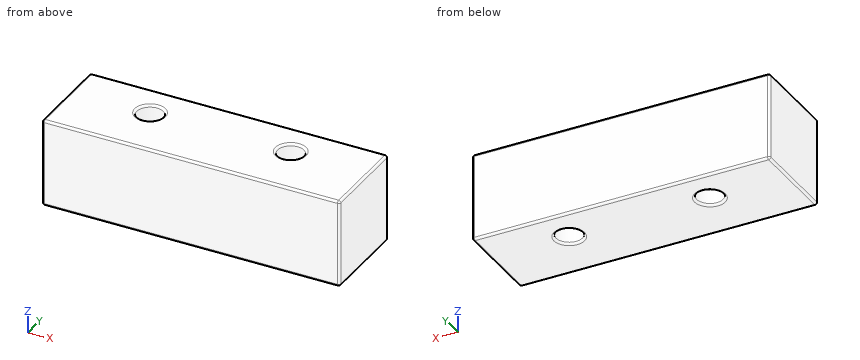
```python
from build123d import *

# Parameters (mm, degrees)
SKETCH1_W           = 67.684274796
SKETCH1_H           = 20.635526277
SKETCH1_R           = 3
BOSS_EXTRUDE1_DEPTH = 20
FILLET1_R           = 0.5


with BuildPart() as part:
    # Sketch1 → Boss-Extrude1 (new body)
    with BuildSketch(Plane.XY):
        with Locations((-33.842137398, 10.317763139)):
            Rectangle(SKETCH1_W, SKETCH1_H)
        with Locations((-49.842137398, 12.635526277)):
            Circle(SKETCH1_R, mode=Mode.SUBTRACT)
        with Locations((-17.842137398, 12.635526277)):
            Circle(SKETCH1_R, mode=Mode.SUBTRACT)
    extrude(amount=BOSS_EXTRUDE1_DEPTH)

    # Fillet1
    fillet1_edges = [part.edges().sort_by_distance(p)[0] for p in [
        (-52.842137398, 12.635526277, 0),
        (-52.842137398, 12.635526277, 20),
        (-33.842137398, 20.635526277, 20),
        (-20.842137398, 12.635526277, 0),
        (-20.842137398, 12.635526277, 20),
        (-67.684274796, 10.317763139, 20),
        (-33.842137398, 0, 20),
        (-67.684274796, 10.317763139, 0),
        (-33.842137398, 20.635526277, 0),
        (0, 10.317763139, 0),
        (-33.842137398, 0, 0),
        (-67.684274796, 0, 10),
        (-67.684274796, 20.635526277, 10),
        (0, 20.635526277, 10),
        (0, 0, 10),
        (0, 10.317763139, 20),
    ]]
    fillet(fillet1_edges, radius=FILLET1_R)


solid = part.part
```
Source: CAD feature listing. Evaluate the final solid. Frame: model axes, mm. Give positions to 0.01 mm unless a question says otherwise; leave off trailing zeros. Order: outer loops, then holes, each group sorted by start corner. A loop starts at its lowest first (then second) coordinate and runs counter-clockwise, first axis right, second up.
(1) Contact query for a flat-ended pin moving along its axis: P1, Ø5, axis at x = -49.84, y = 12.64, coming from the -Z side. Output: stop coordinate, or through.
(2) Material intervals for line 1 along X through (y, z) = (12.75, 2.25); line 2 along X through (y, z) = (10, 17.75); line 3 along Y through (x, z) = (-20, 3.5), sorted ascending.
(3) Section query A-A (z = 15.25). Return the cut outline in (x, y).
Outcome:
1. P1: passes through
2. line 1: x = -67.68 to -52.84, -46.84 to -20.84, -14.84 to 0
2. line 2: x = -67.68 to -51.28, -48.41 to -19.28, -16.41 to 0
2. line 3: y = 0 to 10.55, 14.72 to 20.64
3. outline: (-67.68, 0.5) arc R0.5 ccw to (-67.18, 0) - (-0.5, 0) arc R0.5 ccw to (0, 0.5) - (0, 20.14) arc R0.5 ccw to (-0.5, 20.64) - (-67.18, 20.64) arc R0.5 ccw to (-67.68, 20.14) - close; hole circle Ø6 at (-49.84, 12.64); hole circle Ø6 at (-17.84, 12.64)
